```python
from build123d import *

# Parameters (mm, degrees)
SKETCH1_R           = 25.4
BOSS_EXTRUDE1_DEPTH = 6
SKETCH2_R           = 10
SKETCH3_R           = 1.5
CUT_EXTRUDE1_DEPTH  = 11.4


with BuildPart() as part:
    # Sketch1 → Boss-Extrude1 (new body)
    with BuildSketch(Plane.XY):
        Circle(SKETCH1_R)
    extrude(amount=BOSS_EXTRUDE1_DEPTH)

    # Sketch2 → Cut-Revolve1 (revolve, cut)
    with BuildSketch(Plane(origin=(0, 0, 0), x_dir=(0, 0, -1), z_dir=(1, 0, 0))):
        with Locations((-13, 25.4)):
            Circle(SKETCH2_R)
    revolve(axis=Axis((0, 0, 6), (0, 0, -1)), mode=Mode.SUBTRACT)

    # Mirror1: part across plane


with BuildPart() as part_1:
    add(part.part)
    add(part.part.mirror(Plane.XY))

    # Sketch3 → Cut-Extrude1 (cut, through all)
    with BuildSketch(Plane(origin=(0, 15, 0), x_dir=(1, 0, 0), z_dir=(0, 1, 0))):
        Circle(SKETCH3_R)
    extrude(amount=CUT_EXTRUDE1_DEPTH, mode=Mode.SUBTRACT)


solid = part_1.part
```
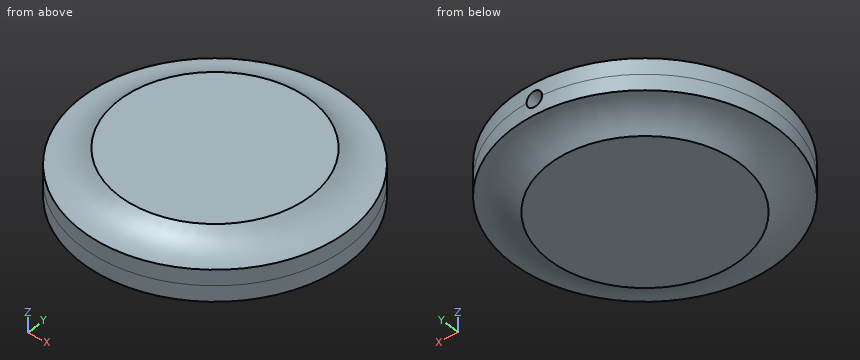
Geometry: final body of the model. Coordinates: model frame, mm. Round coordinates to 2 decimals unless told otherwise and drop trailing zeros. Order: outer loops, then holes, each group sorted by start corner. A loop starts at its lowest first (then second) coordinate and runs counter-clockwise, first axis right, second up. Notation, with made-up numbers: M 7.5,76 L 14.5,76 A27 cw 14.5,114 Z; hole C 77.5,16 d5. An arc over 180 degrees is marked long. One line per item, written item: value.
(1) Pin query (flat end, axial travel): P1, Ø5, axis at x = 19.5, z = 2.5, coming from the -Y side; P2, Ø4, axis at y = 1, z = 3.5, coming from the -X side; P3, Ø4, axis at x = -8.5, z = -0.5, coming from the -Y side; P4, Ø1.5, axis at x = 19.5, z = 0.5, coming from the +Y side. Return the tip coordinate at first contact, or that it passes through.
Result sheet:
P1: y = -18.87
P2: x = -25.4
P3: y = -24.55
P4: y = 17.13
(2) Cut plane D-D (z = 4.25). Return the cut outline in (x, y), and give its area (3 significant figures).
Result sheet:
outline: C 0,0 d41.12
area: 1,330 mm2
(3) Cut plane B-B (y = 0). Return the cut outline in (x, z), and give its area (4 significant figures).
Result sheet:
outline: M -25.4,-3 A10 cw -18.26,-6 L 18.26,-6 A10 cw 25.4,-3 L 25.4,3 A10 cw 18.26,6 L -18.26,6 A10 cw -25.4,3 Z
area: 550.5 mm2
(4) Cut plane A-A (x = 0). Return the cut outline in (y, z).
Result sheet:
outline: M -25.4,-3 A10 cw -18.26,-6 L 18.26,-6 A10 cw 25.4,-3 L 25.4,-1.5 L 15,-1.5 L 15,1.5 L 25.4,1.5 L 25.4,3 A10 cw 18.26,6 L -18.26,6 A10 cw -25.4,3 Z
(5) Line query: probe 1 along Z at (x, y) = (0, 17.75); probe 2 along X at (y, z) = (18.5, 0); probe 3 along X at (y, z) = (22, 0). Output: solid intervals per line, ascending. Write a range as [from, to].
Result sheet:
probe 1: [-6, -1.5], [1.5, 6]
probe 2: [-17.4, -1.5], [1.5, 17.4]
probe 3: [-12.69, -1.5], [1.5, 12.69]
(6) Cut plane C-C (z = -0.75). Return the cut outline in (x, y).
Result sheet:
outline: M -1.3,15 L -1.3,25.37 A25.4 ccw long 1.3,25.37 L 1.3,15 Z
